```python
from build123d import *

# Parameters (mm, degrees)
SKETCH2_R               = 1
BOSS_EXTRUDE2_DEPTH     = 30
CUT_EXTRUDE1_DEPTH      = 37.224991373
CUT_EXTRUDE1_DEPTH_BACK = 37.224991373
SKETCH3_R               = 2.15
SKETCH3_W               = 10
SKETCH3_H               = 7


with BuildPart() as part:
    # Sketch2 → Boss-Extrude2 (new body)
    with BuildSketch(Plane.XY):
        with BuildLine():
            Line((1, 3.5), (1, 20))
            Line((1, 20), (2.5, 20))
            Line((2.5, 20), (2.5, 0))
            ThreePointArc((2.5, 0), (-1.767766953, -1.767766953), (0, 2.5))
            ThreePointArc((0, 2.5), (0.707106781, 2.792893219), (1, 3.5))
        make_face()
        Circle(SKETCH2_R, mode=Mode.SUBTRACT)
    extrude(amount=BOSS_EXTRUDE2_DEPTH)

    # Sketch3 → Cut-Extrude1 (cut, two sides: drawn at the far end of the back side and taken through both)
    with BuildSketch(Plane.ZY.offset(-1).offset(-CUT_EXTRUDE1_DEPTH_BACK)):
        with Locations(Location((7.5, 15.5, 0), (0, 0, 270))):
            Circle(SKETCH3_R)
        with Locations(Location((22.5, 15.5, 0), (0, 0, 270))):
            Circle(SKETCH3_R)
        with Locations((15, 0)):
            Rectangle(SKETCH3_W, SKETCH3_H)
    extrude(amount=CUT_EXTRUDE1_DEPTH + CUT_EXTRUDE1_DEPTH_BACK, mode=Mode.SUBTRACT)


solid = part.part
```
Build history of the part. All positions in model axes, mm. A direction names the side the tool comes from. Round coordinates to 2 decimals unless told otherwise and drop trailing zeros. Write each loop counter-clockwise with the first axis right and the second up, starting at its lowest first coordinate (ties: lowest second). Pieces come first, ordered by that corner, then holes.
1) Band-saw the part on A-A, the plane z = 22.5. List the corners of the cut face in (x, y).
2) Band-saw the part on B-B, the plane z = 27. List the corners of the cut face in (x, y).
3) Drill centre lines: probe 1 along X at (y, z) = (0, 6.25); probe 2 along X at (y, z) = (6.75, 21.75); probe 3 along Y at (x, z) = (-0.3, 28.5). Where is each one in solid material? Low to high.
4) Pin check, flat tips, straight feed: pin 1 (5.5 mm diameter, centred on y = 15.5, z = 7.5, fed in from -X); pin 2 (1.2 mm diameter, centred on x = 1.5, z = 15.5, fed in from -Y); pin 3 (1.6 mm diameter, centred on x = 0, y = 0, fed in from -Z); pin 4 (2 mm diameter, centred on x = -1, z = 22, fed in from +Y). Stop position of each tip, or through.
5) 3-axis set-ups, long thin cutter, end or side, ignore diameter. For faces 1 (the flat face through (1, 12, 15)), 2 (the flat face through (2, 20, 15)), 3 (the flat face through (1, 1, 10)): which of +Z, -Z, +X, -X, +Y, -Y reach the whole face in a straight line?
6) Band-saw the part on D-D, the plane y = 10.5. List the corners of the cut face in (x, z).
7) Band-saw the part on C-C, the plane x = -1.9. List the corners of the cut face in (y, z).
8) Mould opens along Z. For faces 4 (the flat face through (2, 6, 0)), 5 (the cylindrical face through (0.699, 2.785, 4.93)), 6 (the cylindrical face through (1.76, 14.51, 20.59)) say: +Z half, -Z half, draft (parallel to the pull), parting line (faces both ways), or undercut.
Ans:
1. outline: (0, 2.5) arc R2.5 ccw (long way) to (2.5, 0) - (2.5, 13.35) - (1, 13.35) - (1, 3.5) arc R1 cw to start; (1, 17.65) - (2.5, 17.65) - (2.5, 20) - (1, 20) - close; hole circle Ø2 at (0, 0)
2. outline: (0, 2.5) arc R2.5 ccw (long way) to (2.5, 0) - (2.5, 20) - (1, 20) - (1, 3.5) arc R1 cw to start; hole circle Ø2 at (0, 0)
3. probe 1: x = -2.5 to -1, 1 to 2.5
3. probe 2: x = 1 to 2.5
3. probe 3: y = -2.48 to -0.95, 0.95 to 2.48
4. pin 1: stops at x = 1
4. pin 2: stops at y = 3.5
4. pin 3: passes through
4. pin 4: stops at y = 2.5
5. face 1: +Z, -Z, -X, +Y
5. face 2: +Z, -Z, +X, -X, +Y
5. face 3: +X, -X, -Y
6. outline: (1, 0) - (2.5, 0) - (2.5, 30) - (1, 30) - close
7. outline: (-1.62, 0) - (1.62, 0) - (1.62, 10) - (-1.62, 10) - close; (-1.62, 20) - (1.62, 20) - (1.62, 30) - (-1.62, 30) - close
8. face 4: -Z half
8. face 5: draft
8. face 6: undercut
